Part model, mm, in its own coordinate system. Coordinates: 2 decimals unless noted, no trailing zeros. Order: outer loops, then holes, each group sorted by start corner. A loop starts at its lowest first (then second) coordinate and runs counter-clockwise, first axis right, second up.
1) Wall check: L1, parallel to Z at x = 99.54, y = 1.6; L2, parallel to X at y = 1.4, z = -11.98; L3, parallel to X at y = 1.45, z = -8.5. Give the ranges that are in metal, low to high.
2) Cut at A-A (x = 5.46). List the corners of the cut face in (y, z), and give its area (3 significant figures).
3) Pin check, flat tip, straight feed: pin 1 Ø1.8 at (x, z) = (99.54, -11.98) entering from -Y. Stop position of the tip, or through.
```python
from build123d import *

# Parameters (mm, degrees)
SKETCH1_W                = 105
SKETCH1_H                = 90
BOSS_EXTRUDE1_DEPTH      = 2
M3_CLEARANCE_HOLE1_D     = 3
M3_CLEARANCE_HOLE1_DEPTH = 2
M3_CLEARANCE_HOLE1_TIP   = 0.901290929
SKETCH4_W                = 4
SKETCH4_H                = 3
CUT_EXTRUDE1_DEPTH       = 139.307628134
FILLET1_R                = 1
FILLET2_R                = 1
FILLET3_R                = 1
FILLET4_R                = 1
LPATTERN1_COUNT          = 2
LPATTERN1_PITCH          = 75
LPATTERN1_COUNT_DIR2     = 3
LPATTERN1_PITCH_DIR2     = 38
FILLET1_OF_LPATTERN1_R   = 1
FILLET2_OF_LPATTERN1_R   = 1
FILLET3_OF_LPATTERN1_R   = 1
FILLET4_OF_LPATTERN1_R   = 1


with BuildPart() as part:
    # Sketch1 → Boss-Extrude1 (new body)
    with BuildSketch(Plane(origin=(0, 0, 0), x_dir=(1, 0, 0), z_dir=(0, 1, 0))):
        with Locations((52.5, 45)):
            Rectangle(SKETCH1_W, SKETCH1_H)
    extrude(amount=BOSS_EXTRUDE1_DEPTH)

    # M3 Clearance Hole1
    with Locations(Plane(origin=(0, 2, 0), x_dir=(1, 0, 0), z_dir=(0, 1, 0))):
        with Locations((5.46, 11.98), (5.46, 78.02), (99.54, 78.02), (99.54, 11.98)):
            Hole(M3_CLEARANCE_HOLE1_D / 2, depth=M3_CLEARANCE_HOLE1_DEPTH)
            with Locations((0, 0, -(M3_CLEARANCE_HOLE1_DEPTH + M3_CLEARANCE_HOLE1_TIP / 2))):  # 118° drill point
                Cone(0, M3_CLEARANCE_HOLE1_D / 2, M3_CLEARANCE_HOLE1_TIP, mode=Mode.SUBTRACT)

    # Sketch4 → Cut-Extrude1 (cut, through all)
    with BuildSketch(Plane(origin=(0, 2, 0), x_dir=(1, 0, 0), z_dir=(0, 1, 0))):
        with Locations((14.5, 82.5)):
            Rectangle(SKETCH4_W, SKETCH4_H)
    cut_extrude1 = extrude(amount=-CUT_EXTRUDE1_DEPTH, mode=Mode.SUBTRACT)

    # Fillet1
    fillet1_edges = [part.edges().sort_by_distance(p)[0] for p in [
        (12.5, 1, -84),
    ]]
    fillet(fillet1_edges, radius=FILLET1_R)

    # Fillet2
    fillet2_edges = [part.edges().sort_by_distance(p)[0] for p in [
        (12.5, 1, -81),
    ]]
    fillet(fillet2_edges, radius=FILLET2_R)

    # Fillet3
    fillet3_edges = [part.edges().sort_by_distance(p)[0] for p in [
        (16.5, 1, -84),
    ]]
    fillet(fillet3_edges, radius=FILLET3_R)

    # Fillet4
    fillet4_edges = [part.edges().sort_by_distance(p)[0] for p in [
        (16.5, 1, -81),
    ]]
    fillet(fillet4_edges, radius=FILLET4_R)

    # LPattern1: Cut-Extrude1 2 × 3
    with Locations(*[(j * LPATTERN1_PITCH_DIR2, 0, i * LPATTERN1_PITCH) for i in range(LPATTERN1_COUNT) for j in range(LPATTERN1_COUNT_DIR2) if (i, j) != (0, 0)]):
        add(cut_extrude1, mode=Mode.SUBTRACT)

    # Fillet1 of LPattern1
    fillet1_of_lpattern1_edges = [part.edges().sort_by_distance(p)[0] for p in [
        (50.5, 1, -84),
        (88.5, 1, -84),
        (12.5, 1, -9),
        (50.5, 1, -9),
        (88.5, 1, -9),
    ]]
    fillet(fillet1_of_lpattern1_edges, radius=FILLET1_OF_LPATTERN1_R)

    # Fillet2 of LPattern1
    fillet2_of_lpattern1_edges = [part.edges().sort_by_distance(p)[0] for p in [
        (50.5, 1, -81),
        (88.5, 1, -81),
        (12.5, 1, -6),
        (50.5, 1, -6),
        (88.5, 1, -6),
    ]]
    fillet(fillet2_of_lpattern1_edges, radius=FILLET2_OF_LPATTERN1_R)

    # Fillet3 of LPattern1
    fillet3_of_lpattern1_edges = [part.edges().sort_by_distance(p)[0] for p in [
        (54.5, 1, -84),
        (92.5, 1, -84),
        (16.5, 1, -9),
        (54.5, 1, -9),
        (92.5, 1, -9),
    ]]
    fillet(fillet3_of_lpattern1_edges, radius=FILLET3_OF_LPATTERN1_R)

    # Fillet4 of LPattern1
    fillet4_of_lpattern1_edges = [part.edges().sort_by_distance(p)[0] for p in [
        (54.5, 1, -81),
        (92.5, 1, -81),
        (16.5, 1, -6),
        (54.5, 1, -6),
        (92.5, 1, -6),
    ]]
    fillet(fillet4_of_lpattern1_edges, radius=FILLET4_OF_LPATTERN1_R)


solid = part.part
```
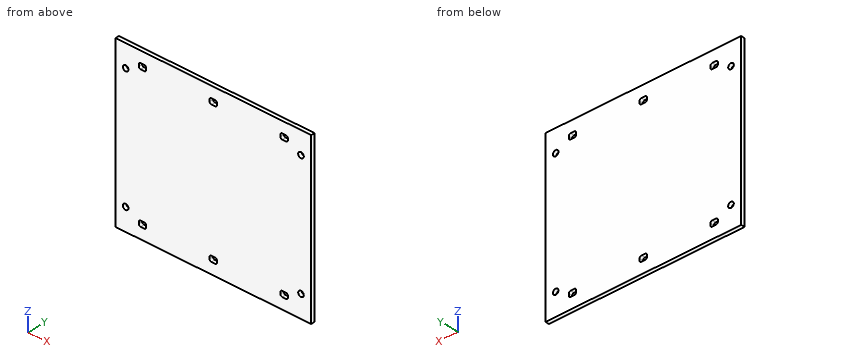
Geometry check:
1. L1: z = -90 to -79.52, -76.52 to -13.48, -10.48 to 0
1. L2: x = 0 to 3.96, 6.96 to 98.04, 101.04 to 105
1. L3: x = 0 to 12.63, 16.37 to 50.63, 54.37 to 88.63, 92.37 to 105
2. outline: (0, -90) - (2, -90) - (2, -79.52) - (0, -79.52) - close; (0, -76.52) - (2, -76.52) - (2, -13.48) - (0, -13.48) - close; (0, -10.48) - (2, -10.48) - (2, 0) - (0, 0) - close
2. area: 168 mm2
3. pin 1: passes through
